For this review, take the finished solid that the model builds, in its own axes (mm). A direction names the side the tool comes from. Round coordinates to 2 decimals unless told otherwise and drop trailing zeros. Order: outer loops, then holes, each group sorted by start corner. A loop starts at its lowest first (then second) coordinate and runs counter-clockwise, first axis right, second up. Notation, with made-up numbers: M -36.75,60.25 L 16.25,60.25 A19 ccw 16.25,83.25 Z; hole C 46.5,-14 d10. An arc over 180 degrees is marked long. Put each result on its own line as item: value.
Autodesk Inventor part; units mm, degrees
ref_plane "YZ Plane" through (0, 0, 0) normal (1, 0, 0) x (0, 1, 0)
ref_plane "XZ Plane" through (0, 0, 0) normal (0, 1, 0) x (-1, 0, 0)
ref_plane "XY Plane" through (0, 0, 0) normal (0, 0, 1) x (1, 0, 0)
sketch "Sketch1" plane through (0, 0, 0) normal (0, 1, 0) x (-1, 0, 0)
  line L0 (9.6647, -7.8359) -> (-9.6647, -7.8359)
  line L1 (-9.6647, -7.8359) -> (-9.6647, 7.8359)
  line L2 (-9.6647, 7.8359) -> (9.6647, 7.8359)
  line L3 (9.6647, 7.8359) -> (9.6647, -7.8359)
  point P0 (0, 0)
  point P1 (-9.6647, 0)
  point P2 (0, -7.8359)
  dimension "d0" = 19.3294
  dimension "d1" = 15.6718
extrude "Extrusion1" add sketch "Sketch1" along normal blind 1.5367
sketch "Sketch2" plane through (0, 1.5367, 0) normal (0, 1, 0) x (1, 0, 0)
  line L0 (-2.5654, -3.0925) -> (2.5654, -3.0925)
  line L1 (2.5654, -3.0925) -> (2.5654, 3.0925)
  line L2 (2.5654, 3.0925) -> (-2.5654, 3.0925)
  line L3 (-2.5654, 3.0925) -> (-2.5654, -3.0925)
  point P0 (0, 0)
  point P1 (-2.5654, 0)
  point P2 (0, 3.0925)
  dimension "d4" = 5.1308
  dimension "d5" = 6.1849
extrude "Extrusion2" add sketch "Sketch2" along normal blind 9.7028
sketch "Sketch3" plane through (0, 0, 0) normal (0, -1, 0) x (1, 0, 0)
  circle A0 centre (51.2064, 25.6032) radius 0.8001
  circle A1 centre (6.4897, 3.556) radius 0.8001
  circle A2 centre (6.4897, 0) radius 0.8001
  circle A3 centre (6.4897, -3.556) radius 0.8001
  line L0 (9.6647, 7.8359) -> (9.6647, -7.8359)
  point P0 (0, 0)
  dimension "d8" = 1.6002
  dimension "d9" = 1.6002
  dimension "d10" = 1.6002
  dimension "d11" = 7.112
  dimension "d12" = 3.556
  dimension "d13" = 3.175
  dimension "d14" = 3.175
extrude "Extrusion3" add sketch "Sketch3" along normal blind 2.54 contours A1 | A2 | A3
properties part number "IF Remote reader"
(1) For faces 1 (the face through (5.855, -1.252, 4.043)), 2 (the face through (-2.565, 6, 0)), 3 (the face through (0, 6, -3.092)), list the 3-axis set-ups (+Z, -Z, +X, -X, +Y, -Y) from which the entire face can be reached by the end or side of a thin tool; tool diameter is ignored.
A:
face 1: -Y
face 2: +Z, -Z, -X, +Y
face 3: -Z, +X, -X, +Y
(2) Add section C-C on y = 6. Give the boundary of the cut face in (x, z), then the cut area to 3 significant figures.
A:
outline: M -2.57,-3.09 L 2.57,-3.09 L 2.57,3.09 L -2.57,3.09 Z
area: 31.7 mm2
(3) Add section B-B on z = 0. Give the boundary of the cut face in (x, y), then the cut area to 3 significant figures.
A:
outline: M -9.66,0 L 5.69,0 L 5.69,-2.54 L 7.29,-2.54 L 7.29,0 L 9.66,0 L 9.66,1.54 L 2.57,1.54 L 2.57,11.24 L -2.57,11.24 L -2.57,1.54 L -9.66,1.54 Z
area: 83.6 mm2
(4) To check wall thickness, follow L1, parallel to Y at x = 2.25, z = 3.5; L2, parallel to X at y = 4.5, z = 2.75; L3, parallel to Z at x = -2, y = 4.5. State the ranges of each line that lie inside material, in increasing order.
A:
L1: y = 0 to 1.54
L2: x = -2.57 to 2.57
L3: z = -3.09 to 3.09
(5) Add section D-D on z = 2.5. Give the boundary of the cut face in (x, y), then the cut area to 3 significant figures.
A:
outline: M -9.66,0 L 9.66,0 L 9.66,1.54 L 2.57,1.54 L 2.57,11.24 L -2.57,11.24 L -2.57,1.54 L -9.66,1.54 Z
area: 79.5 mm2
(6) Insertion check: pin 1 Ø6 at (x, y) = (-7.5, 4.5) entering from +Z; pin 2 Ø2 at (y, z) = (3.5, -2.5) entering from -X; pin 3 Ø1.5 at (x, z) = (-1, 5.5) entering from -Y; pin 4 Ø4 at (x, y) = (-0.5, 8) entering from -Z. Each pin has a flat end and moves straight along its axis. Give the tip position at first contact, or say it passes through.
A:
pin 1: stops at z = 7.84
pin 2: stops at x = -2.57
pin 3: stops at y = 0
pin 4: stops at z = -3.09
(7) Draft analysis for pull direction Z (two halves, no side actions). For faces 4 (the face through (0, 6, 3.092)), 5 (the face through (5.69, -1.25, -0.04)), 6 (the face through (2.565, 6, 0)), state which applies: released by +Z, released by -Z, zero draft, split by the parting line, or undercut.
A:
face 4: released by +Z
face 5: undercut
face 6: zero draft
(8) Add section A-A on x = -1.25. Give the boundary of the cut face in (y, z).
A:
outline: M 0,-7.84 L 1.54,-7.84 L 1.54,-3.09 L 11.24,-3.09 L 11.24,3.09 L 1.54,3.09 L 1.54,7.84 L 0,7.84 Z
